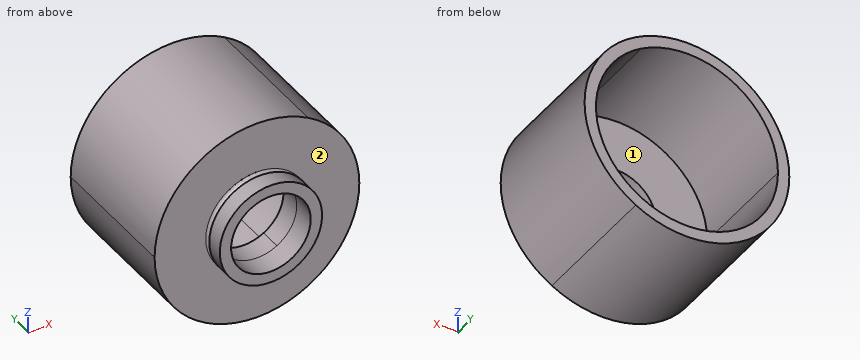
Autodesk Inventor part; units mm, degrees
ref_plane "XZ Plane" through (0, 0, 0) normal (0, 1, 0) x (-1, 0, 0)
ref_plane "XY Plane" through (0, 0, 0) normal (0, 0, 1) x (1, 0, 0)
sketch "スケッチ6" plane through (0, 0, 0) normal (0, 1, 0) x (-1, 0, 0)
  arc A0 (9, 0) -> (-4.5, 7.7942) centre (0, 0) ccw
  line L0 (0, 0) -> (-4.5, 7.7942) construction
  line L1 (0, 0) -> (9, 0) construction
  arc A1 (8, 0) -> (-4, 6.9282) centre (0, 0) ccw
  line L2 (0, 0) -> (-4, 6.9282) construction
  line L3 (0, 0) -> (8, 0) construction
  arc A2 (7, 0) -> (-3.5, 6.0622) centre (0, 0) ccw
  line L4 (0, 0) -> (-3.5, 6.0622) construction
  line L5 (0, 0) -> (7, 0) construction
  arc A3 (4.7, 0) -> (-2.35, 4.0703) centre (0, 0) ccw
  arc A4 (3.5, 0) -> (-1.75, 3.0311) centre (0, 0) ccw
  line L6 (4.5041, 1.3429) -> (6.7082, 2)
  arc A5 (10.9533, 0) -> (5.4767, 9.4859) centre (0, 0) ccw
  line L7 (0, 0) -> (5.4767, 9.4859) construction
  line L8 (0, 0) -> (10.9533, 0) construction
  line L9 (-1.0891, 4.5721) -> (-1.6221, 6.8095)
  line L10 (0, 0) -> (9, 0)
  line L11 (0, 0) -> (-4.5, 7.7942)
  point P0 (-1.6221, 6.8095)
  point P1 (-4, 6.9282)
  point P2 (-1.75, 3.0311)
  dimension "d33" = 9
  dimension "d34" = 120
  dimension "d35" = 120
  dimension "d36" = 1
  dimension "d37" = 120
  dimension "d38" = 2
  dimension "d39" = 4.7
  dimension "d40" = 3.5
  dimension "d41" = 2
  dimension "d42" = 60
extrude "押し出し6" add sketch "スケッチ6" along normal blind 1.9 contours L10 A2 L11 A1 | L10 A3 L6 A2 | A2 L9 A3 L11 | L6 A3 L9 A2 | L10 A4 L11 A3
sketch "スケッチ7" plane through (0, 0, 0) normal (0, -1, 0) x (1, 0, 0)
  arc A0 (4, 6.9282) -> (-8, 0) centre (0, 0) ccw
  arc A1 (4.5, 7.7942) -> (-9, 0) centre (0, 0) ccw
  arc A2 (4, 6.9282) -> (-8, 0) centre (0, 0) ccw
  line L0 (0, 0) -> (4, 6.9282) construction
  line L1 (0, 0) -> (-8, 0) construction
  line L2 (4.5, 7.7942) -> (4, 6.9282)
  line L3 (-9, 0) -> (-8, 0)
  dimension "d45" = 120
  dimension "d46" = 9
  dimension "d47" = 8
  dimension "d48" = 120
extrude "押し出し7" add sketch "スケッチ7" against normal blind 12
pattern_circular "円形状パターン1" count 3 over 360 about axis through (0, 0, 0) along (0, 1, 0)
sketch "スケッチ9" plane through (0, 0, 0) normal (0, -1, 0) x (1, 0, 0)
  circle A0 centre (0, 0) radius 4.5
  circle A1 centre (0, 0) radius 3.5
  dimension "d62" = 9
extrude "押し出し9" add sketch "スケッチ9" along normal blind 2
sketch "スケッチ11" plane through (0, 0, 0) normal (1, 0, 0) x (0, 1, 0)
  line L0 (0, 4.5) -> (-2, 4.5)
  circle A0 centre (-0.25, 4.5) radius 0.25
  line L1 (0, 9) -> (0, -9)
  point P0 (0, 0)
  point P1 (-0.5, 4.5)
  dimension "d73" = 0.5
sketch3d "3D スケッチ1"
  arc A0 (4.5, 0, 0) -> (0, 0, -4.5) centre (0, 0, 0) ccw
  arc A1 (0, 0, -4.5) -> (-4.5, 0, 0) centre (0, 0, 0) ccw
  arc A2 (-4.5, 0, 0) -> (0, 0, 4.5) centre (0, 0, 0) ccw
  arc A3 (0, 0, 4.5) -> (4.5, 0, 0) centre (0, 0, 0) ccw
sweep "スイープ1" cut profiles "スケッチ11" path "3D スケッチ1" picked at (-0.194, 4.3148) contours A0 L0
properties part number "wheel" material "ABS プラスチック"
Input: part model. Units: mm. Frame: model coordinates. Face numbers are marked on the shaded views. Give positions to 0.01 mm unless a question says otherwise; leave off trailing zeros. Order: outer loops, then holes, each group sorted by start corner. A loop starts at its lowest first (then second) coordinate and runs counter-clockwise, first axis right, second up. Notation, with made-up numbers: M 69,89 L 104,89 A34 ccw 104,128 Z; hole C 70.25,79 d9. An arc over 180 degrees is marked long. Answer as a JSON object with one key per item and string values.
1. Cut plane C-C, the plane x = -7.5. Output: boundary loops of the cut face in (y, z), and give its area (3 significant figures).
Result sheet:
{"outline": "M 0,-4.97 L 12,-4.97 L 12,-2.78 L 1.9,-2.78 L 1.9,2.78 L 12,2.78 L 12,4.97 L 0,4.97 Z", "area": "63.2 mm²"}
2. Ray query, line 1 (X direction, y = -0.55, z = 0); line 2 (Y direction, x = 5.75, z = 2). Return the intervals inside material, ascending. Write a range as [from, to].
Result sheet:
{"line 1": "[-4.5, -3.5], [3.5, 4.5]", "line 2": "[0, 1.9]"}
3. First-contact query: P1, Ø4, axis at x = -6.5, y = 1, coming from the -Z side; P2, Ø2, axis at x = -7, z = 4, coming from the -Y side; P3, Ø3, axis at x = -4.5, y = 0, coming from the -Z side. Flat tips, straight axial feed; report the tip coordinate or a pass-through.
Result sheet:
{"P1": "z = -7.79", "P2": "y = 0", "P3": "z = -8.49"}
4. Cut plane B-B, the plane y = 3. Output: boundary loops of the cut face in (x, z), and give its area (3 significant figures).
Result sheet:
{"outline": "M -9,0 A9 ccw 4.5,-7.79 A9 ccw 4.5,7.79 A9 ccw Z; hole M -8,0 A8 ccw 4,-6.93 A8 ccw 4,6.93 A8 ccw Z", "area": "53.4 mm²"}
5. Pull-direction query (Z, two-part tool) for the marked faces 1 and 2; classes: +Z half, -Z half, draft (parallel to the pull), parting line (faces both ways), or undercut.
Result sheet:
{"face 1": "undercut", "face 2": "draft"}
6. Cut plane A-A, the plane x = 0. Output: boundary loops of the cut face in (y, z).
Result sheet:
{"outline": "M -2,-4.5 L -0.5,-4.5 A0.25 cw 0,-4.5 L 0,-9 L 12,-9 L 12,-8 L 1.9,-8 L 1.9,-3.5 L -2,-3.5 Z; M -2,3.5 L 1.9,3.5 L 1.9,8 L 12,8 L 12,9 L 0,9 L 0,4.5 A0.25 cw -0.5,4.5 L -2,4.5 Z"}
7. Cut plane D-D, the plane y = 1. Output: boundary loops of the cut face in (x, z).
Result sheet:
{"outline": "M -9,0 A9 ccw 4.5,-7.79 A9 ccw 4.5,7.79 A9 ccw Z; hole M -3.5,0 A3.5 ccw 1.75,-3.03 A3.5 ccw 1.75,3.03 A3.5 ccw Z"}
